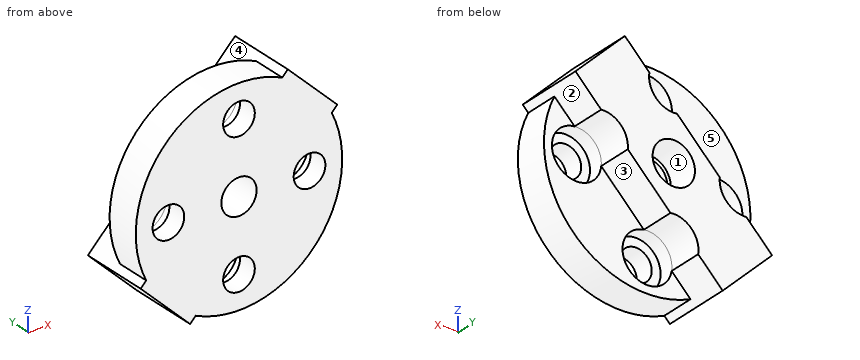
```python
from build123d import *

# Parameters (mm, degrees)
SKETCH1_R           = 18.57375
SKETCH1_R_2         = 2.85115
BOSS_EXTRUDE1_DEPTH = 6.1849
BOSS_EXTRUDE2_DEPTH = 12.4714
SKETCH3_R           = 4.445
CUT_EXTRUDE1_DEPTH  = 2.667
CIRPATTERN1_COUNT   = 4
SKETCH4_R           = 3.81
CUT_EXTRUDE2_DEPTH  = 5.715
SKETCH5_R           = 3.175
CUT_EXTRUDE3_DEPTH  = 7.7564


with BuildPart() as part:
    # Sketch1 → Boss-Extrude1 (new body)
    with BuildSketch(Plane(origin=(0, 0, 0), x_dir=(1, 0, 0), z_dir=(0, 1, 0))):
        Circle(SKETCH1_R)
        with Locations((0, 12.7)):
            Circle(SKETCH1_R_2, mode=Mode.SUBTRACT)
        with Locations((-12.7, 0)):
            Circle(SKETCH1_R_2, mode=Mode.SUBTRACT)
        with Locations((0, -12.7)):
            Circle(SKETCH1_R_2, mode=Mode.SUBTRACT)
        with Locations((12.7, 0)):
            Circle(SKETCH1_R_2, mode=Mode.SUBTRACT)
    extrude(amount=BOSS_EXTRUDE1_DEPTH)

    # Sketch2 → Boss-Extrude2 (add)
    with BuildSketch(Plane(origin=(0, 0, 0), x_dir=(1, 0, 0), z_dir=(0, 1, 0))):
        with BuildLine():
            Line((-8.797939445, 17.874031217), (-4.392677204, 13.380008809))
            ThreePointArc((-4.392677204, 13.380008809), (-3.174280479, 9.588413838), (0.592258402, 8.294633388))
            Line((0.592258402, 8.294633388), (8.278225813, 0.453803969))
            ThreePointArc((8.278225813, 0.453803969), (9.525719521, -3.111586162), (13.065518202, -4.429945987))
            Line((13.065518202, -4.429945987), (17.694994159, -9.152699719))
            Line((17.694994159, -9.152699719), (8.797939445, -17.874031217))
            Line((8.797939445, -17.874031217), (4.392677204, -13.380008809))
            ThreePointArc((4.392677204, -13.380008809), (3.174280479, -9.588413838), (-0.592258402, -8.294633388))
            Line((-0.592258402, -8.294633388), (-8.278225813, -0.453803969))
            ThreePointArc((-8.278225813, -0.453803969), (-9.525719521, 3.111586162), (-13.065518202, 4.429945987))
            Line((-13.065518202, 4.429945987), (-17.694994159, 9.152699719))
            Line((-17.694994159, 9.152699719), (-8.797939445, 17.874031217))
        make_face()
    extrude(amount=BOSS_EXTRUDE2_DEPTH)

    # Sketch3 → Cut-Extrude1 (cut)
    with BuildSketch(Plane(origin=(0, 6.1849, 0), x_dir=(1, 0, 0), z_dir=(0, 1, 0))):
        with Locations((0, -12.7)):
            Circle(SKETCH3_R)
    cut_extrude1 = extrude(amount=-CUT_EXTRUDE1_DEPTH, mode=Mode.SUBTRACT)

    # CirPattern1: Cut-Extrude1 ×4 about axis
    cirpattern1_axis = Axis((0, 6.1849, 0), (0, -1, 0))
    for i in range(1, CIRPATTERN1_COUNT):
        add(cut_extrude1.rotate(cirpattern1_axis, i * 360 / CIRPATTERN1_COUNT), mode=Mode.SUBTRACT)

    # Sketch4 → Cut-Extrude2 (cut)
    with BuildSketch(Plane(origin=(0, 12.4714, 0), x_dir=(1, 0, 0), z_dir=(0, 1, 0))):
        Circle(SKETCH4_R)
    extrude(amount=-CUT_EXTRUDE2_DEPTH, mode=Mode.SUBTRACT)

    # Sketch5 → Cut-Extrude3 (cut, through all)
    with BuildSketch(Plane(origin=(0, 6.7564, 0), x_dir=(1, 0, 0), z_dir=(0, 1, 0))):
        Circle(SKETCH5_R)
    extrude(amount=-CUT_EXTRUDE3_DEPTH, mode=Mode.SUBTRACT)


solid = part.part
```
Source: CAD feature listing. Evaluate the final solid. Frame: model axes, mm. Face numbers are marked on the shaded views. A direction names the side the tool comes from. Round coordinates to 2 decimals unless told otherwise and drop trailing zeros. Order: outer loops, then holes, each group sorted by start corner. A loop starts at its lowest first (then second) coordinate and runs counter-clockwise, first axis right, second up. Notation, with made-up numbers: (-16.5, -17.5) -> (13.5, -17.5) arc R15 cw to (13.5, -8.5) -> close; hole circle Ø11 at (27.5, -2). An arc over 180 degrees is marked (long way). One line per item, written item: value. Start each with the question number.
Q1. Section query A-A (x = 0). Return the cut outline in (y, z) (3 decimals).
Q2. Section query B-B (y = 10.5). Return the cut outline in (x, z) (3 decimals).
Q3. Access query for the marked faces 1, 2, 3, 4 and 5. Directions: +Z, -Z, +X, -X, +Y, -Y. A direction counts if a zero-diameter tool reaches every point of the face in a straight line with its end or side. Return the directions, or none.
Q4. Pin query (flat end, axial travel): pin 1 (7 mm diameter, centred on x = 0.5, z = 12.5, fed in from +Y); pin 2 (6 mm diameter, centred on x = 0, z = 0, fed in from +Y) (3 decimals); pin 3 (1.5 mm diameter, centred on y = 11, z = -3, fed in from +X); pin 4 (3 mm diameter, centred on y = 3, z = -4, fed in from +X). Return the tip coordinate at first contact, or that it passes through.
Q5. Material intervals for probe 1 along X at (y, z) = (5.45, 0) (3 decimals); probe 2 along X at (y, z) = (1.3, 0) (3 decimals), sorted ascending.
Q6. Section query D-D (z = 12.7). Return the cut outline in (x, y) (3 decimals), plus the area to 3 significant figures.
Q7. Section query C-C (z = 0). Return the cut outline in (x, y) (3 decimals), plus the area to 3 significant figures.
Findings below:
1. outline: (0, -18.574) -> (6.185, -18.574) -> (6.185, -17.145) -> (3.518, -17.145) -> (3.518, -15.551) -> (0, -15.551) -> close; (0, -9.849) -> (3.518, -9.849) -> (3.518, -8.255) -> (12.471, -8.255) -> (12.471, -3.81) -> (6.756, -3.81) -> (6.756, -3.175) -> (0, -3.175) -> close; (0, 3.175) -> (6.756, 3.175) -> (6.756, 3.81) -> (12.471, 3.81) -> (12.471, 8.255) -> (3.518, 8.255) -> (3.518, 9.849) -> (0, 9.849) -> close; (0, 15.551) -> (3.518, 15.551) -> (3.518, 17.145) -> (6.185, 17.145) -> (6.185, 18.574) -> (0, 18.574) -> close
2. outline: (-17.695, -9.153) -> (-8.798, -17.874) -> (-4.393, -13.38) arc R4.445 cw to (0.592, -8.295) -> (8.278, -0.454) arc R4.445 cw to (13.066, 4.43) -> (17.695, 9.153) -> (8.798, 17.874) -> (4.393, 13.38) arc R4.445 cw to (-0.592, 8.295) -> (-8.278, 0.454) arc R4.445 cw to (-13.066, -4.43) -> close; hole circle Ø7.62 at (0, 0)
3. face 1: +Y
3. face 2: +X, +Y
3. face 3: -Z, +X, +Y
3. face 4: +Z, +Y
3. face 5: +Z, -X, +Y
4. pin 1: y = 3.52
4. pin 2: through
4. pin 3: x = 6.52
4. pin 4: x = 18.4
5. probe 1: -18.574 to -17.145, -8.255 to -3.175, 3.175 to 8.255, 17.145 to 18.574
5. probe 2: -18.574 to -15.551, -9.849 to -3.175, 3.175 to 9.849, 15.551 to 18.574
6. outline: (-13.553, 0) -> (-2.851, 0) -> (-2.851, 3.518) -> (-4.445, 3.518) -> (-4.445, 6.185) -> (-13.553, 6.185) -> close; (2.851, 0) -> (14.076, 0) -> (14.076, 12.471) -> (4.445, 12.471) -> (4.445, 3.518) -> (2.851, 3.518) -> close
6. area: 188 mm²
7. outline: (-18.574, 0) -> (-15.551, 0) -> (-15.551, 3.518) -> (-17.145, 3.518) -> (-17.145, 6.185) -> (-18.574, 6.185) -> close; (-9.849, 0) -> (-3.175, 0) -> (-3.175, 6.756) -> (-3.81, 6.756) -> (-3.81, 12.471) -> (-8.255, 12.471) -> (-8.255, 3.518) -> (-9.849, 3.518) -> close; (3.175, 0) -> (9.849, 0) -> (9.849, 3.518) -> (8.255, 3.518) -> (8.255, 12.471) -> (3.81, 12.471) -> (3.81, 6.756) -> (3.175, 6.756) -> close; (15.551, 0) -> (18.574, 0) -> (18.574, 6.185) -> (17.145, 6.185) -> (17.145, 3.518) -> (15.551, 3.518) -> close
7. area: 160 mm²
